from build123d import *

# Parameters (mm, degrees)
SKETCH_1_R          = 75
EXTRUDE_1_DEPTH     = 3
SKETCH_2_R          = 3
CUT_EXTRUDE_1_DEPTH = 3


with BuildPart() as part:
    # Эскиз1 → Бобышка-Вытянуть1 (new body)
    with BuildSketch(Plane(origin=(0, 0, 0), x_dir=(1, 0, 0), z_dir=(0, 1, 0))):
        with Locations(Location((0, 0, 0), (0, 0, 270))):
            Circle(SKETCH_1_R)
    extrude(amount=EXTRUDE_1_DEPTH)

    # Эскиз2 → Вырез-Вытянуть1 (cut)
    with BuildSketch(Plane(origin=(0, 3, 0), x_dir=(1, 0, 0), z_dir=(0, 1, 0))):
        with Locations(Location((-70, 0, 0), (0, 0, 270))):
            Circle(SKETCH_2_R)
        with Locations(Location((70, 0, 0), (0, 0, 90))):
            Circle(SKETCH_2_R)
        with Locations(Location((0, -70, 0), (0, 0, 270))):
            Circle(SKETCH_2_R)
        with Locations(Location((0, 70, 0), (0, 0, 90))):
            Circle(SKETCH_2_R)
        with Locations(Location((-49.497474683, -49.497474683, 0), (0, 0, 270))):
            Circle(SKETCH_2_R)
        with Locations(Location((-49.497474683, 49.497474683, 0), (0, 0, 90))):
            Circle(SKETCH_2_R)
        with Locations(Location((49.497474683, -49.497474683, 0), (0, 0, 270))):
            Circle(SKETCH_2_R)
        with Locations(Location((49.497474683, 49.497474683, 0), (0, 0, 90))):
            Circle(SKETCH_2_R)
    extrude(amount=-CUT_EXTRUDE_1_DEPTH, mode=Mode.SUBTRACT)


solid = part.part
CAD build for the part. Positions are in the model's coordinates, mm. Coordinates: 2 decimals unless noted, no trailing zeros. Order: outer loops, then holes, each group sorted by start corner. A loop starts at its lowest first (then second) coordinate and runs counter-clockwise, first axis right, second up. Notation, with made-up numbers: (-4.75, 55.5) -> (16.25, 55.5) arc R14 cw to (16.25, 60.5) -> close; hole circle Ø6 at (60, -9). An arc over 180 degrees is marked (long way). Answer in a Markdown table with one row per item.
1) Band-saw the part on B-B (z = 0). List the corners of the cut face in (x, y), and give its area (3 significant figures).
Check values:
| item | result |
|---|---|
| outline | (-75, 0) -> (-73, 0) -> (-73, 3) -> (-75, 3) -> close; (-67, 0) -> (67, 0) -> (67, 3) -> (-67, 3) -> close; (73, 0) -> (75, 0) -> (75, 3) -> (73, 3) -> close |
| area | 414 mm2 |
2) Band-saw the part on D-D (z = -70). List the corners of the cut face in (x, y), and give its area (3 significant figures).
Check values:
| item | result |
|---|---|
| outline | (-26.93, 0) -> (-3, 0) -> (-3, 3) -> (-26.93, 3) -> close; (3, 0) -> (26.93, 0) -> (26.93, 3) -> (3, 3) -> close |
| area | 144 mm2 |
3) Band-saw the part on A-A (x = 0). List the corners of the cut face in (y, z).
Check values:
| item | result |
|---|---|
| outline | (0, -75) -> (3, -75) -> (3, -73) -> (0, -73) -> close; (0, -67) -> (3, -67) -> (3, 67) -> (0, 67) -> close; (0, 73) -> (3, 73) -> (3, 75) -> (0, 75) -> close |
4) Drill centre lines: line 1 (X direction, y = 2.45, z = 0); line 2 (Z direction, x = -2, y = 0.35); line 3 (Z direction, x = -25.5, y = 2.4). Where is each one in solid material? Low to high.
Check values:
| item | result |
|---|---|
| line 1 | -75 to -73, -67 to 67, 73 to 75 |
| line 2 | -74.97 to -72.24, -67.76 to 67.76, 72.24 to 74.97 |
| line 3 | -70.53 to 70.53 |
5) Band-saw the part on C-C (x = 70). List the corners of the cut face in (y, z).
Check values:
| item | result |
|---|---|
| outline | (0, -26.93) -> (3, -26.93) -> (3, -3) -> (0, -3) -> close; (0, 3) -> (3, 3) -> (3, 26.93) -> (0, 26.93) -> close |
6) Flat gauge pins, fed straight in: P1, Ø3.5, axis at x = 70, z = 0, coming from the -Y side; P2, Ø8, axis at x = 49.5, z = 49.5, coming from the -Y side. Where does each tip first touch, or does it go through?
Check values:
| item | result |
|---|---|
| P1 | through |
| P2 | y = 0 |
7) Mould opens along Z. For faces 1 (the face through (-51.3, 1.5, 47.1)), 2 (the face through (1, 0, -1)), 3 (the face through (-45.636, 1.479, -59.517)) say: pulls with the +Z half, pulls with the -Z half, needs draft (parallel to the pull), parting line crosses it, or undercut.
Check values:
| item | result |
|---|---|
| face 1 | undercut |
| face 2 | needs draft |
| face 3 | parting line crosses it |
